Verification items for the finished model (mm, model axes). Give positions to 0.01 mm unless a question says otherwise; leave off trailing zeros. Order: outer loops, then holes, each group sorted by start corner. A loop starts at its lowest first (then second) coordinate and runs counter-clockwise, first axis right, second up.
from build123d import *

# Parameters (mm, degrees)
SKETCH_2_W          = 10
SKETCH_2_H          = 10
SKETCH_2_W_2        = 8
SKETCH_2_H_2        = 8
EXTRUDE_1_DEPTH     = 170
CUT_EXTRUDE_1_REACH = 172.587
SKETCH_3_R          = 2.15
SKETCH_4_R          = 2.15
CUT_EXTRUDE_2_DEPTH = 171.587221092


with BuildPart() as part:
    # ｽｹｯﾁ2 → 押し出し-薄板1 (new body)
    with BuildSketch(Plane(origin=(0, 0, 0), x_dir=(0, 0, -1), z_dir=(1, 0, 0))):
        with Locations((5, 5)):
            Rectangle(SKETCH_2_W, SKETCH_2_H)
        with Locations((5, 5)):
            Rectangle(SKETCH_2_W_2, SKETCH_2_H_2, mode=Mode.SUBTRACT)
    extrude(amount=EXTRUDE_1_DEPTH)

    # ｶｯﾄ - 押し出し1: up to this face of the body (flat: up to its plane)
    cut_extrude_1_end = Plane(part.part.faces().sort_by_distance((85, 0, -5))[0])
    # ｽｹｯﾁ3 → ｶｯﾄ - 押し出し1 (cut, up to the picked face)
    with BuildSketch(Plane(origin=(0, 10, 0), x_dir=(1, 0, 0), z_dir=(0, 1, 0)), mode=Mode.PRIVATE) as cut_extrude_1_sk1:
        with Locations(Location((14, 5, 0), (0, 0, 270))):
            Circle(SKETCH_3_R)
    cut_extrude_1_tool1 = split(extrude(cut_extrude_1_sk1.sketch, amount=-CUT_EXTRUDE_1_REACH, mode=Mode.PRIVATE), bisect_by=cut_extrude_1_end, keep=Keep.BOTH, mode=Mode.PRIVATE)
    # ｽｹｯﾁ3 → ｶｯﾄ - 押し出し1 (cut, up to the picked face)
    with BuildSketch(Plane(origin=(0, 10, 0), x_dir=(1, 0, 0), z_dir=(0, 1, 0)), mode=Mode.PRIVATE) as cut_extrude_1_sk2:
        with Locations(Location((34, 5, 0), (0, 0, 270))):
            Circle(SKETCH_3_R)
    cut_extrude_1_tool2 = split(extrude(cut_extrude_1_sk2.sketch, amount=-CUT_EXTRUDE_1_REACH, mode=Mode.PRIVATE), bisect_by=cut_extrude_1_end, keep=Keep.BOTH, mode=Mode.PRIVATE)
    # ｽｹｯﾁ3 → ｶｯﾄ - 押し出し1 (cut, up to the picked face)
    with BuildSketch(Plane(origin=(0, 10, 0), x_dir=(1, 0, 0), z_dir=(0, 1, 0)), mode=Mode.PRIVATE) as cut_extrude_1_sk3:
        with Locations(Location((136, 5, 0), (0, 0, 90))):
            Circle(SKETCH_3_R)
    cut_extrude_1_tool3 = split(extrude(cut_extrude_1_sk3.sketch, amount=-CUT_EXTRUDE_1_REACH, mode=Mode.PRIVATE), bisect_by=cut_extrude_1_end, keep=Keep.BOTH, mode=Mode.PRIVATE)
    # ｽｹｯﾁ3 → ｶｯﾄ - 押し出し1 (cut, up to the picked face)
    with BuildSketch(Plane(origin=(0, 10, 0), x_dir=(1, 0, 0), z_dir=(0, 1, 0)), mode=Mode.PRIVATE) as cut_extrude_1_sk4:
        with Locations(Location((156, 5, 0), (0, 0, 90))):
            Circle(SKETCH_3_R)
    cut_extrude_1_tool4 = split(extrude(cut_extrude_1_sk4.sketch, amount=-CUT_EXTRUDE_1_REACH, mode=Mode.PRIVATE), bisect_by=cut_extrude_1_end, keep=Keep.BOTH, mode=Mode.PRIVATE)
    add(cut_extrude_1_tool1.solids().sort_by(Axis((14, 10, -5), (0, -1, 0)))[0], mode=Mode.SUBTRACT)
    add(cut_extrude_1_tool2.solids().sort_by(Axis((34, 10, -5), (0, -1, 0)))[0], mode=Mode.SUBTRACT)
    add(cut_extrude_1_tool3.solids().sort_by(Axis((136, 10, -5), (0, -1, 0)))[0], mode=Mode.SUBTRACT)
    add(cut_extrude_1_tool4.solids().sort_by(Axis((156, 10, -5), (0, -1, 0)))[0], mode=Mode.SUBTRACT)

    # ｽｹｯﾁ4 → ｶｯﾄ - 押し出し2 (cut, through all)
    with BuildSketch(Plane.XY):
        with Locations((105, 5)):
            Circle(SKETCH_4_R)
        with Locations((85, 5)):
            Circle(SKETCH_4_R)
        with Locations((65, 5)):
            Circle(SKETCH_4_R)
    extrude(amount=-CUT_EXTRUDE_2_DEPTH, mode=Mode.SUBTRACT)


solid = part.part
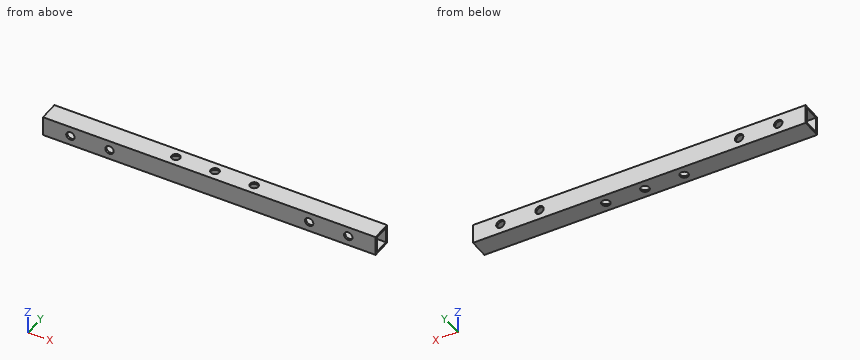
(1) Scan lines: line 1 (X direction, y = 9.2, z = -5); line 2 (Z direction, x = 109.5, y = 4.25); line 3 (Y direction, x = 22.5, z = -7.25). Record each from-to range of solid material in increasing order.
Solved:
line 1: x = 0 to 11.85, 16.15 to 31.85, 36.15 to 133.85, 138.15 to 153.85, 158.15 to 170
line 2: z = -10 to -9, -1 to 0
line 3: y = 0 to 1, 9 to 10
(2) Section check A-A, the plane x = 136. Enter the section's corners in (y, z).
Solved:
outline: (0, -10) - (10, -10) - (10, -7.15) - (9, -7.15) - (9, -9) - (1, -9) - (1, -7.15) - (0, -7.15) - close; (0, -2.85) - (1, -2.85) - (1, -1) - (9, -1) - (9, -2.85) - (10, -2.85) - (10, 0) - (0, 0) - close
(3) Section check B-B, the plane y = 5. Give the number of separate pieces and of enclosed holes in the cut face, then the cut area to 3 significant figures.
Solved:
separate pieces: 8
enclosed holes: 0
area: 314 mm2
(4) Go/stop test with a flat-tipped pin: pin 1 (4 mm diameter, centred on x = 136, z = -5, fed in from -Y). Record where the tip stops, or that it passes through.
Solved:
pin 1: passes through
(5) Section check C-C, the plane x = 58. Enter the section's corners in (y, z).
Solved:
outline: (0, -10) - (10, -10) - (10, 0) - (0, 0) - close; hole (1, -9) - (9, -9) - (9, -1) - (1, -1) - close
